Design review of the part built by this model. Coordinates are the model's own, in mm. Coordinates: 2 decimals unless noted, no trailing zeros. Write each loop counter-clockwise with the first axis right and the second up, starting at its lowest first coordinate (ties: lowest second). Pieces come first, ordered by that corner, then holes. Notation, with made-up numbers: M -39,52.5 L -25,52.5 A11 ccw -25,56.5 Z; hole C 73,68.25 d6. An arc over 180 degrees is marked long. Write item = value, one per line.
```python
from build123d import *

# Parameters (mm, degrees)
F3_D     = 13
F3_DEPTH = 50
F3_TIP   = 3.9055940237
F4_R     = 5


with BuildPart() as f1:
    # F0 (on Front) → F1 (revolve)
    with BuildSketch(Plane.XZ):
        Polygon((-12.7, -45.7867538678), (0, -45.7867538678), (0, 94.2131613321), (-7, 94.2131613321), (-12.7, 54.2132461322), align=None)
    revolve(axis=Axis((0, 0, 24.2132037321), (0, 0, 1)))

    # F3
    with Locations(Plane.XY.offset(94.2131613321)):
        with Locations((0, 0)):
            Hole(F3_D / 2, depth=F3_DEPTH)
            with Locations((0, 0, -(F3_DEPTH + F3_TIP / 2))):  # 118° drill point
                Cone(0, F3_D / 2, F3_TIP, mode=Mode.SUBTRACT)

    # F4
    f4_edges = [f1.edges().sort_by_distance(p)[0] for p in [
        (12.7, 0, -45.786754),
    ]]
    fillet(f4_edges, radius=F4_R)


solid = f1.part
```
Q1. Consider section B-B, the plane z = 78. State the section outline as (x, y) points, and give its area (3 significant figures).
Check result:
outline = C 0,0 d18.62; hole C 0,0 d13
area = 140 mm²
Q2. The part is to be moulded in two halves that separate along X. For faces 1 (the conical face through (-9.433, -2.971, 73.933)), 2 (the flat face through (0, 0, -45.787)), 3 (the conical face through (-0.9, -0.69, 40.99)), 4 (the cylindrical face through (5.158, -3.955, 68.863)), say which applies: +X half, -X half, draft (parallel to the pull), parting line (faces both ways), or undercut.
Check result:
face_1 = parting line
face_2 = draft
face_3 = undercut
face_4 = undercut
Q3. Consider section A-A, the plane z = -27.5. State the section outline as (x, y) points, and give its area (3 significant figures).
Check result:
outline = C 0,0 d25.4
area = 507 mm²
Q4. Wall thickness on line 1 (X direction, y = 0, z = 84.5); line 2 (X direction, y = 0, z = 69.5); line 3 (Y direction, x = 0, z = 82): over which ranges is each line inside the solid? List them lowest first.
Check result:
line_1 = -8.38 to -6.5, 6.5 to 8.38
line_2 = -10.52 to -6.5, 6.5 to 10.52
line_3 = -8.74 to -6.5, 6.5 to 8.74
Q5. For P1, Ø10, axis at y = -7.5, z = 15.5, coming from the +X side; P2, Ø5, axis at x = -4, z = -20, coming from the -Y side; P3, Ø12, axis at x = -7.5, z = -8, coming from the +Y side, all flat-tipped, find the tip position at first contact; note any pin that passes through.
Check result:
P1 = 12.45
P2 = -12.61
P3 = 12.61
